Could you check a few things on this model? Use its own coordinates, in mm. A direction names the side the tool comes from. Coordinates: 2 decimals unless noted, no trailing zeros. Loops run counter-clockwise (first coordinate to the right, second up) from the corner with the lowest first, then second, coordinate; pieces in that order, holes last.
from build123d import *

# Parameters (mm, degrees)
SKETCH1_W           = 50
SKETCH1_H           = 66.15
SKETCH1_R           = 11
SKETCH1_R_2         = 1.55
BOSS_EXTRUDE1_DEPTH = 4
SKETCH2_W           = 50
SKETCH2_H           = 4
BOSS_EXTRUDE2_DEPTH = 38
SKETCH3_R           = 1.5
CUT_EXTRUDE1_DEPTH  = 78.017027338
CHAMFER1_SIZE       = 10
CHAMFER1_SIZE2      = 4.663076582


with BuildPart() as part:
    # Sketch1 → Boss-Extrude1 (new body)
    with BuildSketch(Plane(origin=(0, 0, 0), x_dir=(0, 0, -1), z_dir=(1, 0, 0))):
        Rectangle(SKETCH1_W, SKETCH1_H)
        with Locations((0, 11.925)):
            Circle(SKETCH1_R, mode=Mode.SUBTRACT)
        with Locations((-15.5, 27.425)):
            Circle(SKETCH1_R_2, mode=Mode.SUBTRACT)
        with Locations((15.5, 27.425)):
            Circle(SKETCH1_R_2, mode=Mode.SUBTRACT)
        with Locations((15.5, -3.575)):
            Circle(SKETCH1_R_2, mode=Mode.SUBTRACT)
        with Locations((-15.5, -3.575)):
            Circle(SKETCH1_R_2, mode=Mode.SUBTRACT)
    extrude(amount=BOSS_EXTRUDE1_DEPTH)

    # Sketch2 → Boss-Extrude2 (add)
    with BuildSketch(Plane.ZY):
        with Locations((0, -31.075)):
            Rectangle(SKETCH2_W, SKETCH2_H)
    extrude(amount=BOSS_EXTRUDE2_DEPTH)

    # Sketch3 → Cut-Extrude1 (cut, through all)
    with BuildSketch(Plane(origin=(0, -29.075, 0), x_dir=(1, 0, 0), z_dir=(0, 1, 0))):
        with Locations(Location((-33, -15, 0), (0, 0, 270))):
            Circle(SKETCH3_R)
        with Locations(Location((-8, -15, 0), (0, 0, 270))):
            Circle(SKETCH3_R)
        with Locations(Location((-8, 15, 0), (0, 0, 90))):
            Circle(SKETCH3_R)
        with Locations(Location((-33, 15, 0), (0, 0, 90))):
            Circle(SKETCH3_R)
    extrude(amount=-CUT_EXTRUDE1_DEPTH, mode=Mode.SUBTRACT)

    # Chamfer1
    chamfer1_edges = [part.edges().sort_by_distance(p)[0] for p in [
        (0, -29.075, 0),
    ]]
    chamfer1_side = [part.faces().sort_by_distance(p)[0] for p in [
        (0, 0.490102601, 0),
    ]]
    chamfer(chamfer1_edges, length=CHAMFER1_SIZE, length2=CHAMFER1_SIZE2, reference=chamfer1_side[0])


solid = part.part
(1) Imagine slicing it at C-C, the plane y = 3. Write out the boundary of the cut face in (x, z), and give its area (3 significant figures).
Answers:
outline: (0, -25) - (4, -25) - (4, -6.43) - (0, -6.43) - close; (0, 6.43) - (4, 6.43) - (4, 25) - (0, 25) - close
area: 149 mm2
(2) Which directions (+Z, -Z, +X, -X, +Y, -Y) give clear straight access to the entire face, cutting with the end or side of a thin tool? Please do faces 4 (the face through (-21, -29.075, 0)), 5 (the face through (-8.9, -31, 13.8)).
Answers:
face 4: +Z, -Z, -X, +Y
face 5: +Y, -Y
(3) Imagine slicing it at B-B, the plane z = 0. Write out the boundary of the cut face in (x, y) (3 decimals).
Answers:
outline: (-38, -33.075) - (4, -33.075) - (4, 0.925) - (0, 0.925) - (0, -19.075) - (-4.663, -29.075) - (-38, -29.075) - close; (0, 22.925) - (4, 22.925) - (4, 33.075) - (0, 33.075) - close
(4) Imagine slicing it at A-A, the plane x = -33. Write out the boundary of the cut face in (y, z) (3 decimals), and give its area (3 significant figures).
Answers:
outline: (-33.075, -25) - (-29.075, -25) - (-29.075, -16.5) - (-33.075, -16.5) - close; (-33.075, -13.5) - (-29.075, -13.5) - (-29.075, 13.5) - (-33.075, 13.5) - close; (-33.075, 16.5) - (-29.075, 16.5) - (-29.075, 25) - (-33.075, 25) - close
area: 176 mm2
(5) Imagine slicing it at D-D, the plane z = -20.5. Write out the boundary of the cut face in (x, y) (3 decimals), and give its area (3 significant figures).
Answers:
outline: (-38, -33.075) - (4, -33.075) - (4, 33.075) - (0, 33.075) - (0, -19.075) - (-4.663, -29.075) - (-38, -29.075) - close
area: 440 mm2
(6) We'd pull the mould along Y, two halves only. Please class faces 1 (the face through (-17, -33.075, 0)), 2 (the face through (-38, -31, 0)), 3 (the face through (1.97, -3.51, 17.05)): +Y half, -Y half, draft (parallel to the pull), parting line (faces both ways), or undercut.
Answers:
face 1: -Y half
face 2: draft
face 3: undercut
(7) For pin 1 (10 mm diameter, centred on y = -12.5, z = -10, fed in from -X); pin 2 (3 mm diameter, centred on x = -25, z = -18, fed in from +Y) (3 decimals); pin 3 (2.5 mm diameter, centred on y = 27.425, z = 15.5, fed in from -X); pin 4 (1.5 mm diameter, centred on y = -25.5, z = 19, fed in from -X), each with a flat end and sliding along its axis, tell me the tip position at first contact or that it passes through.
Answers:
pin 1: stops at x = 0
pin 2: stops at y = -29.075
pin 3: passes through
pin 4: stops at x = -3.35
(8) I need wall thicknesses on probe 1 along Y at (x, z) = (0.8, 15.5) (3 decimals); probe 2 along X at (y, z) = (-30, -15); probe 3 along X at (y, z) = (-2, 8). Which ranges of each line are inside material? Lowest first, please.
Answers:
probe 1: y = -33.075 to -5.125, -2.025 to 25.875, 28.975 to 33.075
probe 2: x = -38 to -34.5, -31.5 to -9.5, -6.5 to 4
probe 3: x = 0 to 4
